```python
from build123d import *

# Parameters (mm, degrees)
SKETCH1_W           = 30
SKETCH1_H           = 50
BOSS_EXTRUDE1_DEPTH = 10
SKETCH2_W           = 5
SKETCH2_H           = 50
BOSS_EXTRUDE2_DEPTH = 5
SKETCH3_R           = 1.625
CUT_EXTRUDE1_DEPTH  = 33.787192622
SKETCH4_R           = 2.7
CUT_EXTRUDE2_DEPTH  = 1.45
CHAMFER1_SIZE       = 2
CHAMFER2_SIZE       = 2
FILLET1_R           = 2
FILLET2_R           = 2
CUT_EXTRUDE6_DEPTH  = 1


with BuildPart() as part:
    # Sketch1 → Boss-Extrude1 (new body)
    with BuildSketch(Plane(origin=(0, 0, 0), x_dir=(1, 0, 0), z_dir=(0, 1, 0))):
        Rectangle(SKETCH1_W, SKETCH1_H)
    extrude(amount=BOSS_EXTRUDE1_DEPTH)

    # Sketch2 → Boss-Extrude2 (add)
    with BuildSketch(Plane(origin=(0, 10, 0), x_dir=(1, 0, 0), z_dir=(0, 1, 0))):
        Rectangle(SKETCH2_W, SKETCH2_H)
    extrude(amount=BOSS_EXTRUDE2_DEPTH)

    # Sketch3 → Cut-Extrude1 (cut, through all)
    with BuildSketch(Plane.XZ):
        with Locations(Location((-12.56, 15, 0), (0, 0, 270))):
            Circle(SKETCH3_R)
        with Locations(Location((-12.56, -15, 0), (0, 0, 270))):
            Circle(SKETCH3_R)
        with Locations(Location((12.56, -15, 0), (0, 0, 270))):
            Circle(SKETCH3_R)
        with Locations(Location((12.56, 15, 0), (0, 0, 270))):
            Circle(SKETCH3_R)
    extrude(amount=-CUT_EXTRUDE1_DEPTH, mode=Mode.SUBTRACT)

    # Sketch4 → Cut-Extrude2 (cut)
    with BuildSketch(Plane.XZ):
        with Locations((-12.56, 15)):
            Circle(SKETCH4_R)
        with Locations((-12.56, -15)):
            Circle(SKETCH4_R)
        with Locations((12.56, -15)):
            Circle(SKETCH4_R)
        with Locations((12.56, 15)):
            Circle(SKETCH4_R)
    extrude(amount=-CUT_EXTRUDE2_DEPTH, mode=Mode.SUBTRACT)

    # Chamfer1
    # the kernel refuses this chamfer: 2 mm, written as the material it takes off along each edge
    with BuildSketch(Plane(origin=(-15, 0, -30.143365976), x_dir=(0.9996219169112968, -0.027495876610586365, 0), z_dir=(0, 0, 1)), Plane(origin=(-15, 0, 11.012661705), x_dir=(0.9996219169112968, -0.027495876610586365, 0), z_dir=(0, 0, 1))) as chamfer1_piece_1:
        Polygon((CHAMFER1_SIZE * 0.999621916911, CHAMFER1_SIZE * 0.0274958766106), (-CHAMFER1_SIZE * 0.0274958766106, CHAMFER1_SIZE * 0.999621916911), (0, 0), align=None)
    extrude(amount=19.130704271, mode=Mode.SUBTRACT)
    with BuildSketch(Plane(origin=(-15, 0, -18.987338295), x_dir=(0.9996219169112968, -0.027495876610586365, 0), z_dir=(0, 0, 1))) as chamfer1_piece_2:
        Polygon((CHAMFER1_SIZE * 0.999621916911, CHAMFER1_SIZE * 0.0274958766106), (-CHAMFER1_SIZE * 0.0274958766106, CHAMFER1_SIZE * 0.999621916911), (0, 0), align=None)
    extrude(amount=37.974676589, mode=Mode.SUBTRACT)

    # Chamfer2
    # the kernel refuses this chamfer: 2 mm, written as the material it takes off along each edge
    with BuildSketch(Plane(origin=(15, 0, 30.143365976), x_dir=(0.027495876610586494, 0.9996219169112968, 0), z_dir=(0, 0, -1)), Plane(origin=(15, 0, -11.012661705), x_dir=(0.027495876610586494, 0.9996219169112968, 0), z_dir=(0, 0, -1))) as chamfer2_piece_1:
        Polygon((CHAMFER2_SIZE * 0.999621916911, -CHAMFER2_SIZE * 0.0274958766106), (-CHAMFER2_SIZE * 0.0274958766106, -CHAMFER2_SIZE * 0.999621916911), (0, 0), align=None)
    extrude(amount=19.130704271, mode=Mode.SUBTRACT)
    with BuildSketch(Plane(origin=(15, 0, 18.987338295), x_dir=(0.027495876610586494, 0.9996219169112968, 0), z_dir=(0, 0, -1))) as chamfer2_piece_2:
        Polygon((CHAMFER2_SIZE * 0.999621916911, -CHAMFER2_SIZE * 0.0274958766106), (-CHAMFER2_SIZE * 0.0274958766106, -CHAMFER2_SIZE * 0.999621916911), (0, 0), align=None)
    extrude(amount=37.974676589, mode=Mode.SUBTRACT)

    # Fillet1
    fillet1_edges = [part.edges().sort_by_distance(p)[0] for p in [
        (-14, 1, 25),
        (-15, 6, 25),
        (-8.75, 10, 25),
        (-2.5, 12.5, 25),
        (0, 15, 25),
        (2.5, 12.5, 25),
        (8.75, 10, 25),
        (15, 6, 25),
        (14, 1, 25),
        (0, 0, 25),
    ]]
    fillet(fillet1_edges, radius=FILLET1_R)

    # Fillet2
    fillet2_edges = [part.edges().sort_by_distance(p)[0] for p in [
        (8.75, 10, -25),
        (2.5, 12.5, -25),
        (0, 15, -25),
        (-2.5, 12.5, -25),
        (-8.75, 10, -25),
        (-15, 6, -25),
        (-14, 1, -25),
        (0, 0, -25),
        (14, 1, -25),
        (15, 6, -25),
    ]]
    fillet(fillet2_edges, radius=FILLET2_R)

    # Mobious Logo → Cut-Extrude6 (cut)
    with BuildSketch(Plane.XZ):
        Polygon((-3.725461883, 6.377557531), (-4.828839221, 6.377557531), (-8.812218423, -0.467122224), (-2.322863572, -0.467122224), (-2.907811009, 0.678144172), (-7.12910045, 0.678144172), align=None)
        Polygon((-3.931176302, 2.917815032), (-3.42624091, 3.740672707), (-0.209615451, -1.888421846), (-8.569101382, -1.888421846), (-8.816410096, -0.785044508), (-1.698296177, -0.785044508), align=None)
        Polygon((-6.549359815, 1.01028133), (-3.42624091, 6.209245734), (0.127008143, 0), (3.661555886, 6.209245734), (6.636670117, 1.01028133), (5.573474433, 1.01028133), (3.661555886, 4.351328327), (0.173638389, -1.77600066), (-3.42624091, 4.514730681), (-5.421111797, 1.01028133), align=None)
        Polygon((3.97947817, 6.377557531), (5.026751575, 6.377557531), (8.972728155, -0.467122224), (2.464671994, -0.467122224), (3.194023116, 0.678144172), (7.252207561, 0.678144172), align=None)
        Polygon((3.661555886, 3.740672707), (0.426229116, -1.888421846), (8.673507182, -1.888421846), (9.111053368, -0.785044508), (1.90363267, -0.785044508), (4.055998695, 2.959823548), align=None)
    extrude(amount=-CUT_EXTRUDE6_DEPTH, mode=Mode.SUBTRACT)


solid = part.part
```
Design review of the part built by this model. Coordinates are the model's own, in mm. A direction names the side the tool comes from. Coordinates: 2 decimals unless noted, no trailing zeros. Order: outer loops, then holes, each group sorted by start corner. A loop starts at its lowest first (then second) coordinate and runs counter-clockwise, first axis right, second up. Notation, with made-up numbers: (53.5, 81.25) - (64.5, 81.25) arc R10 cw to (64.5, 97.25) - close; hole circle Ø10 at (58, 36). An arc over 180 degrees is marked (long way). Answer in a Markdown table with one row per item.
(1) Clearance check with flat-ended pins moving along their axes: pin 1 (3.5 mm diameter, centred on x = -12.56, z = -15, fed in from -Y); pin 2 (1.4 mm diameter, centred on x = 13, z = 15, fed in from -Y); pin 3 (1.5 mm diameter, centred on y = 12, z = 6, fed in from -X); pin 4 (8.5 mm diameter, centred on x = 12.56, z = 15, fed in from +Y). State where each tip first meets the part, or that it passes through.
Checked values:
| item | result |
|---|---|
| pin 1 | y = 1.45 |
| pin 2 | through |
| pin 3 | x = -2.5 |
| pin 4 | y = 10 |
(2) Consider section B-B on y = 4.25. State the section outline as (x, z) points (3 decimals).
Checked values:
| item | result |
|---|---|
| outline | (-15, -23) arc R2 ccw to (-13, -25) - (13, -25) arc R2 ccw to (15, -23) - (15, 23) arc R2 ccw to (13, 25) - (-13, 25) arc R2 ccw to (-15, 23) - close; hole circle Ø3.25 at (-12.56, -15); hole circle Ø3.25 at (-12.56, 15); hole circle Ø3.25 at (12.56, -15); hole circle Ø3.25 at (12.56, 15) |
(3) Consider section C-C on z = -4. State the section outline as (x, y) points.
Checked values:
| item | result |
|---|---|
| outline | (-15, 2) - (-13, 0) - (13, 0) - (15, 2) - (15, 10) - (2.5, 10) - (2.5, 15) - (-2.5, 15) - (-2.5, 10) - (-15, 10) - close |
(4) The part is to be moulded in two halves that separate along Z. For faces 6 (the cylindrical face through (0.18, 0.6, -24.43)), 7 (the flat face through (5.8, 0.5, -0.467)), 8 (the cylindrical face through (-9.86, 0.71, 14.91)), 9 (the cylindrical face through (0.04, 14.65, 24.13)), say which applies: released by +Z, released by -Z, zero draft, split by the parting line, or undercut.
Checked values:
| item | result |
|---|---|
| face 6 | released by -Z |
| face 7 | undercut |
| face 8 | undercut |
| face 9 | released by +Z |
(5) Wall thickness on line 1 along X through (y, z) = (8, 15) (3 decimals); line 2 along X through (y, z) = (5, 14); line 3 along Z through (x, y) = (-1, 0.75): over which ranges is each line inside the solid? List them lowest first. Write a range as from..to.
Checked values:
| item | result |
|---|---|
| line 1 | -15..-14.185, -10.935..10.935, 14.185..15 |
| line 2 | -15..-13.84, -11.28..11.28, 13.84..15 |
| line 3 | -24.56..-1.89, -0.51..0.27, 1.97..24.56 |
(6) For faces 1 (the flat face through (-11, 1.45, -16)), 2 (the cylindrical face through (7.85, 9.43, 24.4)), 3 (the flat face through (-2.5, 12, 0)), 4 (the flat face through (0, 15, 0)), 5 (the flat face through (15, 6, 0)), list the 3-axis set-ups (+Z, -Z, +X, -X, +Y, -Y) from which the entire face can be reached by the end or side of a thin tool; tool diameter is ignored.
Checked values:
| item | result |
|---|---|
| face 1 | -Y |
| face 2 | +Z, +X, +Y |
| face 3 | +Z, -Z, -X, +Y |
| face 4 | +Z, -Z, +X, -X, +Y |
| face 5 | +Z, -Z, +X, +Y, -Y |
(7) Consider section A-A on z = 15. State the section outline as (x, y) points (3 decimals), plus the area to 3 significant figures.
Checked values:
| item | result |
|---|---|
| outline | (-15, 2) - (-14.45, 1.45) - (-14.185, 1.45) - (-14.185, 10) - (-15, 10) - close; (-10.935, 1.45) - (-9.86, 1.45) - (-9.86, 0) - (9.86, 0) - (9.86, 1.45) - (10.935, 1.45) - (10.935, 10) - (2.5, 10) - (2.5, 15) - (-2.5, 15) - (-2.5, 10) - (-10.935, 10) - close; (14.185, 1.45) - (14.45, 1.45) - (15, 2) - (15, 10) - (14.185, 10) - close |
| area | 254 mm^2 |
